```python
from build123d import *

# Parameters (mm, degrees)
F0_R     = 9.5
F0_R_2   = 5
F0_R_3   = 4.1
F1_DEPTH = 1.5
F2_DEPTH = 3.4
F3_DEPTH = 0.6
F4_R     = 1


with BuildPart() as f1:
    # F0 (on Top) → F1 (new body)
    with BuildSketch(Plane.XY):
        Circle(F0_R)
        Circle(F0_R_2, mode=Mode.SUBTRACT)
        Circle(F0_R_2)
        Circle(F0_R_3, mode=Mode.SUBTRACT)
        Circle(F0_R_3)
    extrude(amount=-F1_DEPTH)

    # F0 (on Top) → F2 (join)
    with BuildSketch(Plane.XY):
        Circle(F0_R_3)
    extrude(amount=F2_DEPTH)

    # F0 (on Top) → F3 (join)
    with BuildSketch(Plane.XY):
        Circle(F0_R_2)
        Circle(F0_R_3, mode=Mode.SUBTRACT)
    extrude(amount=F3_DEPTH)

    # F4
    f4_edges = [f1.edges().sort_by_distance(p)[0] for p in [
        (-9.5, 0, 0),
    ]]
    fillet(f4_edges, radius=F4_R)


solid = f1.part
```
Design review of the part built by this model. Coordinates are the model's own, in mm. A direction names the side the tool comes from. Give positions to 0.01 mm unless a question says otherwise; leave off trailing zeros. Order: outer loops, then holes, each group sorted by start corner. A loop starts at its lowest first (then second) coordinate and runs counter-clockwise, first axis right, second up. Notation, with made-up numbers: (79, 12) -> (109, 12) arc R20 ccw to (109, 30) -> close; hole circle Ø9 at (60.5, -20.5). An arc over 180 degrees is marked (long way). Write item = value, one per line. Start each with the question number.
(1) We need section C-C on z = 0.3. Write out the cut boundary in (x, y), plus the area to 3 significant figures.
(2) We need section A-A on x = 0. Write out the cut boundary in (y, z), plus the area to 3 significant figures.
(3) For pin 1 (1 mm diameter, centred on y = -6.5, z = -0.5, fed in from +X); pin 2 (10 mm diameter, centred on x = -2, y = 4, fed in from +Z); pin 3 (2 mm diameter, centred on y = -4, z = -0.5, fed in from -X), all flat-tipped, find the tip position at first contact; note any pin that passes through.
(4) For faces 1 (the face through (0, 0, -1.5)), 2 (the face through (4, -4, 0)), list the 3-axis set-ups (+Z, -Z, +X, -X, +Y, -Y) from which the entire face can be reached by the end or side of a thin tool; tool diameter is ignored.
(5) To check wall thickness, follow line 1 along Z through (x, y) = (1.5, -5.25); line 2 along Z through (x, y) = (-2.5, -4); line 3 along Y through (x, z) = (-3.5, 0.1). State the ranges of each line that lie inside material, in increasing order.
(6) We need section D-D on z = -0.7. Write out the cut boundary in (x, y).
Numbers:
q1.outline = circle Ø10 at (0, 0)
q1.area = 78.5 mm^2
q2.outline = (-9.5, -1.5) -> (9.5, -1.5) -> (9.5, -1) arc R1 ccw to (8.5, 0) -> (5, 0) -> (5, 0.6) -> (4.1, 0.6) -> (4.1, 3.4) -> (-4.1, 3.4) -> (-4.1, 0.6) -> (-5, 0.6) -> (-5, 0) -> (-8.5, 0) arc R1 ccw to (-9.5, -1) -> close
q2.area = 57.0 mm^2
q3.pin_1 = 7.27
q3.pin_2 = 3.4
q3.pin_3 = -8.98
q4.face_1 = -Z, +X, -X, +Y, -Y
q4.face_2 = +Z
q5.line_1 = -1.5 to 0
q5.line_2 = -1.5 to 0.6
q5.line_3 = -3.57 to 3.57
q6.outline = circle Ø18.91 at (0, 0)
